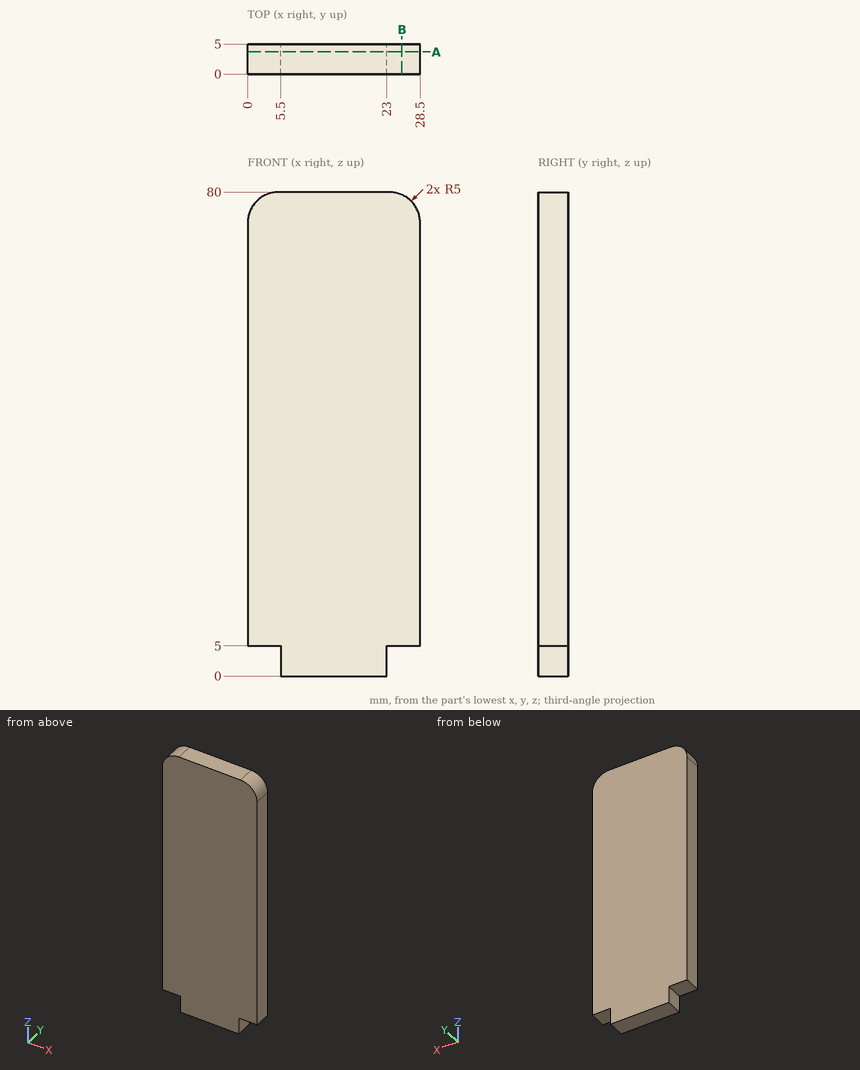
Here's the drawing with two shaded views (mm, measured from the low corner). I have some questions. Give positions to 0.01 mm unless a question says otherwise; leave off trailing zeros. Order: outer loops, then holes, each group sorted by start corner. A loop starts at its lowest first (then second) coordinate and runs counter-clockwise, first axis right, second up.
Q1. Suppose I cut it at A-A, the plane y = 3.7. Write out the boundary of the cut face in (x, z).
Q2. If I drill on line 1 along Z through (x, y) = (23.75, 3.5); line 2 along Z through (x, y) = (26, 2.8); line 3 along X through (y, z) = (3.5, 77.5), over which ranges is the centre line in solid material (lowest first)?
Q3. I'm going to push flat-ended pins straight in: P1, Ø1.5, axis at x = 2, y = 2, coming from the -Z side; P2, Ø2.5, axis at y = 2, z = 2.5, coming from the +X side. Where does each tip first touch, or does it pass through?
Q4. Suppose I cut it at B-B, the plane x = 25.5. Write out the boundary of the cut face in (y, z), and give its area (3 significant figures).
Solution:
1. outline: (0, 5) - (5.5, 5) - (5.5, 0) - (23, 0) - (23, 5) - (28.5, 5) - (28.5, 75) arc R5 ccw to (23.5, 80) - (5, 80) arc R5 ccw to (0, 75) - close
2. line 1: z = 5 to 79.99
2. line 2: z = 5 to 79.33
2. line 3: x = 0.67 to 27.83
3. P1: stops at z = 5
3. P2: stops at x = 23
4. outline: (0, 5) - (5, 5) - (5, 79.58) - (0, 79.58) - close
4. area: 373 mm2
